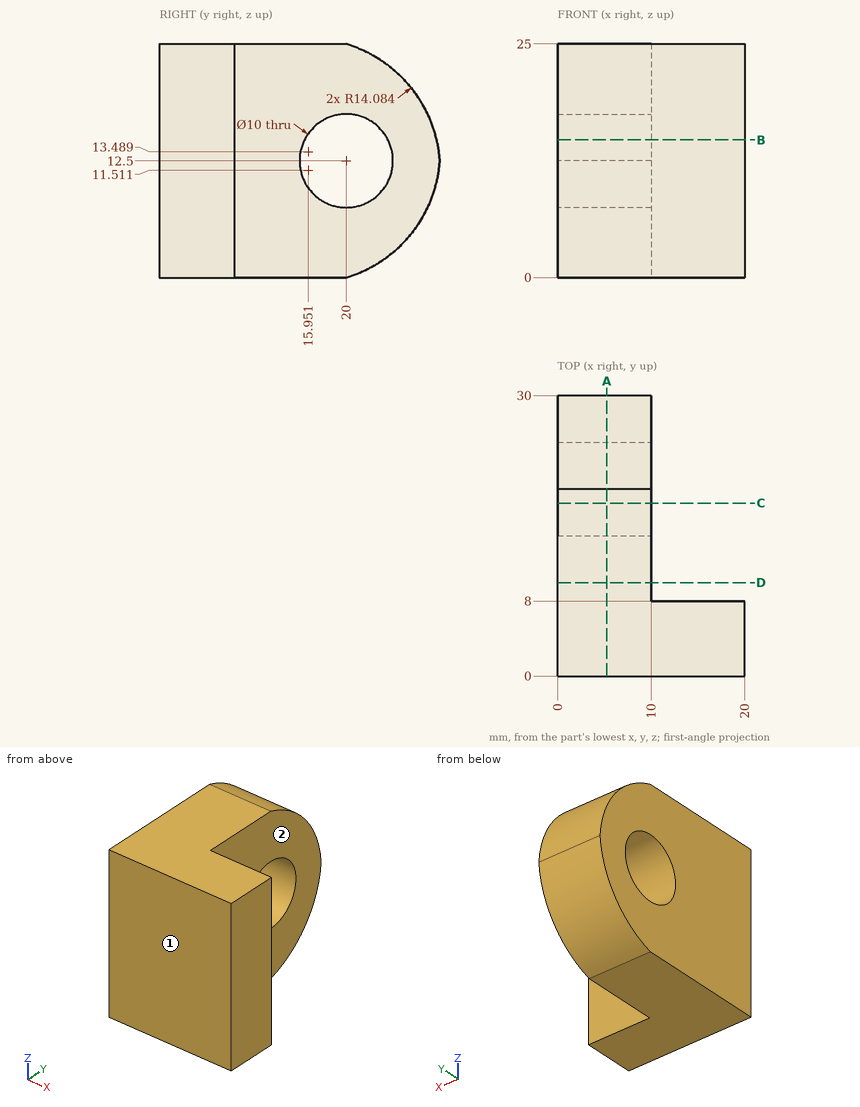
Answer from the drawing. Dimensions are ordinates in mm from the lowest x, y and z of the part. A direction names the side the tool comes from. Give positions to 0.01 mm unless a question says otherwise; leave off trailing zeros. Order: outer loops, then holes, each group sorted by start corner. A loop starts at its lowest first (then second) coordinate and runs counter-clockwise, first axis right, second up. Notation, with made-up numbers: (-6.75, 22) -> (31.25, 22) arc R26 ccw to (31.25, 55) -> close; hole circle Ø10 at (19.25, 18). An arc over 180 degrees is marked (long way). Answer as a JSON object with one key per item and string values. Group by question number.
1. Section C-C on y = 18.5 is taken. Determine the outline of the cut face in (x, z), plus the area to 3 significant figures.
2. Consider line 1 along Y through (x, z) = (6.25, 12.5); line 2 along X through (y, z) = (25.5, 12.5); line 3 along Y through (x, z) = (12.75, 3.5). Determine where each line is inside the solid, lowest interval first. Write a range as [from, to].
3. A tool of negligible diameter and unlimited length cuts with its end or side. For the marked faces 1 and 2, from which of +Z, -Z, +X, -X, +Y, -Y can it reach the whole face along a straight path? Write none if from no direction.
4. Section D-D on y = 10 is taken. Determine the outline of the cut face in (x, z).
5. Section A-A on x = 5.25 is taken. Determine the outline of the cut face in (y, z), plus the area to 3 significant figures.
6. Flat-ended cylindrical pins translate along their axes: pin 1 Ø4 at (y, z) = (12, 11) entering from +X; pin 2 Ø1 at (y, z) = (20, 15) entering from -X; pin 3 Ø8 at (x, z) = (13, 16) entering from +Y. Find the tip coordinate at first contact, or state that the pin passes through.
7. Section B-B on z = 14.75 is taken. Determine the outline of the cut face in (x, y) (1 decimal).
Result sheet:
{
 "1": {"outline": "(0, 0) -> (10, 0) -> (10, 7.73) -> (0, 7.73) -> close; (0, 17.27) -> (10, 17.27) -> (10, 25) -> (0, 25) -> close", "area": "155 mm^2"},
 "2": {"line 1": "y = [0, 15], [25, 30]", "line 2": "x = [0, 10]", "line 3": "y = [0, 8]"},
 "3": {"face 1": "+Z, -Z, +X, -X, -Y", "face 2": "+Z, -Z, +X, +Y"},
 "4": {"outline": "(0, 0) -> (10, 0) -> (10, 25) -> (0, 25) -> close"},
 "5": {"outline": "(0, 0) -> (20, 0) arc R14.08 ccw to (30, 12.5) arc R14.08 ccw to (20, 25) -> (0, 25) -> close; hole circle Ø10 at (20, 12.5)", "area": "601 mm^2"},
 "6": {"pin 1": "stops at x = 10", "pin 2": "passes through", "pin 3": "stops at y = 29.91"},
 "7": {"outline": "(0, 0) -> (20, 0) -> (20, 8) -> (10, 8) -> (10, 15.5) -> (0, 15.5) -> close; (0, 24.5) -> (10, 24.5) -> (10, 29.7) -> (0, 29.7) -> close"}
}
